```python
from build123d import *

# Parameters (mm, degrees)
SKETCH2_R           = 7.5
BOSS_EXTRUDE1_DEPTH = 15
SKETCH3_R           = 3
CUT_EXTRUDE1_DEPTH  = 15
SKETCH4_R           = 5
CUT_EXTRUDE2_DEPTH  = 15
SKETCH5_R           = 7.5
SKETCH5_R_2         = 7
CUT_EXTRUDE3_DEPTH  = 0.5
LPATTERN1_COUNT     = 2
LPATTERN1_PITCH     = 1
LPATTERN2_COUNT     = 2
LPATTERN2_PITCH     = 1
FILLET1_R           = 1


with BuildPart() as part:
    # Sketch2 → Boss-Extrude1 (new, symmetric)
    with BuildSketch(Plane.XY):
        Circle(SKETCH2_R)
    extrude(amount=BOSS_EXTRUDE1_DEPTH, both=True)

    # Sketch3 → Cut-Extrude1 (cut)
    with BuildSketch(Plane.XY.offset(15)):
        Circle(SKETCH3_R)
    extrude(amount=-CUT_EXTRUDE1_DEPTH, mode=Mode.SUBTRACT)

    # Sketch4 → Cut-Extrude2 (cut)
    with BuildSketch(Plane(origin=(0, 0, -15), x_dir=(-1, 0, 0), z_dir=(0, 0, -1))):
        Circle(SKETCH4_R)
    extrude(amount=-CUT_EXTRUDE2_DEPTH, mode=Mode.SUBTRACT)

    # Sketch5 → Cut-Extrude3 (cut)
    with BuildSketch(Plane.XY):
        Circle(SKETCH5_R)
        Circle(SKETCH5_R_2, mode=Mode.SUBTRACT)
    cut_extrude3 = extrude(amount=-CUT_EXTRUDE3_DEPTH, mode=Mode.SUBTRACT)

    # LPattern1: Cut-Extrude3 ×2
    with Locations(*[(0, 0, -i * LPATTERN1_PITCH) for i in range(1, LPATTERN1_COUNT)]):
        add(cut_extrude3, mode=Mode.SUBTRACT)

    # LPattern2: Cut-Extrude3 ×2
    with Locations(*[(0, 0, i * LPATTERN2_PITCH) for i in range(1, LPATTERN2_COUNT)]):
        add(cut_extrude3, mode=Mode.SUBTRACT)

    # Sketch9 → M4 Tapped Hole1 (revolve, cut)
    with BuildSketch(Plane(origin=(-5.303300859, 5.303300859, -9.511136026), x_dir=(-0.7071067811865488, -0.7071067811865464, 0), z_dir=(0, 0, 1))):
        Polygon((0, 0), (0, 6.991420021), (1.65, 6), (1.65, 0), align=None)
    m4_tapped_hole1 = revolve(axis=Axis((-9.793428919, 9.793428919, -9.511136026), (0.7071067811865465, -0.7071067811865487, 0)), mode=Mode.SUBTRACT)

    # Mirror1: M4 Tapped Hole1 across plane
    add(m4_tapped_hole1.mirror(Plane(origin=(0, 0, 0), x_dir=(0, 0, 1), z_dir=(1, 0, 0))), mode=Mode.SUBTRACT)

    # Mirror2: M4 Tapped Hole1 across plane
    add(m4_tapped_hole1.mirror(Plane.XY), mode=Mode.SUBTRACT)

    # Mirror2 copy 1 sketch → Mirror2 copy 1 (revolve, cut)
    with BuildSketch(Plane(origin=(5.303300859, 5.303300859, 9.511136026), x_dir=(0.7071067811865488, -0.7071067811865464, 0), z_dir=(0, 0, -1))):
        Polygon((0, 0), (0, 6.991420021), (1.65, 6), (1.65, 0), align=None)
    revolve(axis=Axis((9.793428919, 9.793428919, 9.511136026), (-0.7071067811865465, -0.7071067811865487, 0)), mode=Mode.SUBTRACT)

    # Fillet1
    fillet1_edges = [part.edges().sort_by_distance(p)[0] for p in [
        (-7.5, 0, -15),
        (-7.5, 0, 15),
    ]]
    fillet(fillet1_edges, radius=FILLET1_R)


solid = part.part
```
Source: CAD feature listing. Evaluate the final solid. Frame: model axes, mm. A direction names the side the tool comes from. Round coordinates to 2 decimals unless told otherwise and drop trailing zeros. Order: outer loops, then holes, each group sorted by start corner. A loop starts at its lowest first (then second) coordinate and runs counter-clockwise, first axis right, second up. Notation, with made-up numbers: (53, 62.25) -> (105, 62.25) arc R6 ccw to (105, 69.25) -> close; hole circle Ø9 at (35, 0.25). An arc over 180 degrees is marked (long way). One line per item, written item: value. Start each with the question number.
Q1. Material intervals for probe 1 along Y at (x, z) = (0, 5.25); probe 2 along Z at (x, y) = (-4.5, 3.5); probe 3 along Y at (x, z) = (0, -9), sorted ascending.
Q2. Pin query (flat end, axial travel): pin 1 (3 mm diameter, centred on y = 4.5, z = 3.5, fed in from -X); pin 2 (8 mm diameter, centred on x = 0.5, y = 2, fed in from -Z); pin 3 (7.5 mm diameter, centred on x = -1, y = 0, fed in from -Z). Return the tip coordinate at first contact, or that it passes through.
Q3. Access query for faces 1 (the flat face through (3, -1, 15)), 2 (the cylindrical face through (-2.307, -4.436, -7.605)), 3 (the flat face through (7, 2, -0.5)). Directions: +Z, -Z, +X, -X, +Y, -Y. A direction counts if a zero-diameter tool reaches every point of the face in a straight line with its end or side. Return the directions, or none.
Q4. Draft query along Z for faces 4 (the cylindrical face through (-7.493, 0.33, 0.254)), 5 (the flat face through (2, -5, -15)), 6 (the flat face through (7, 2, 0.5)). Return one class per face: pulls with the +Z half, pulls with the -Z half, needs draft (parallel to the pull), parting line crosses it, or undercut.
Q5. Section query A-A (z = 13). Return the cut outline in (x, y), plus the area to 3 significant figures.
Q6. Section query B-B (z = -5). Return the cut outline in (x, y).
Findings below:
1. probe 1: -7.5 to -3, 3 to 7.5
1. probe 2: -15 to -11, -8.02 to 8.02, 11 to 15
1. probe 3: -7.5 to -5, 5 to 7.5
2. pin 1: x = -6.87
2. pin 2: z = -15
2. pin 3: z = 0
3. face 1: +Z, +X, -X, +Y, -Y
3. face 2: -Z
3. face 3: none
4. face 4: needs draft
4. face 5: pulls with the -Z half
4. face 6: undercut
5. outline: circle Ø15 at (0, 0); hole circle Ø6 at (0, 0)
5. area: 148 mm²
6. outline: circle Ø15 at (0, 0); hole circle Ø10 at (0, 0)
